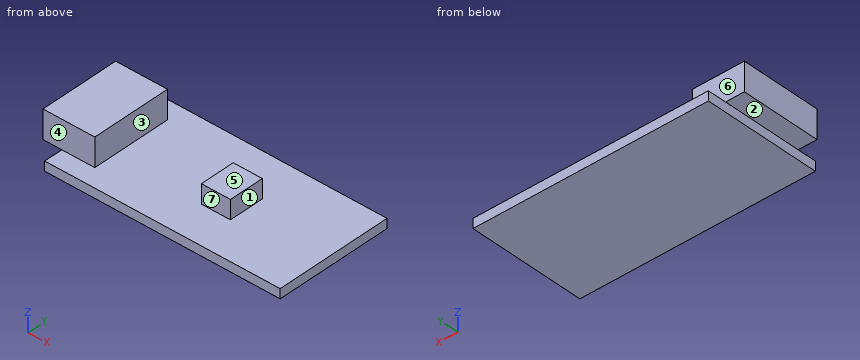
```python
from build123d import *

# Parameters (mm, degrees)
SKIZZE1_W                       = 25
SKIZZE1_H                       = 12.5
SKIZZE1_W_2                     = 3.091607018
SKIZZE1_H_2                     = 3.725771618
AUFSATZ_LINEAR_AUSTRAGEN1_DEPTH = 1
SKIZZE1_2_W                     = 3.091607018
SKIZZE1_2_H                     = 3.725771618
AUFSATZ_LINEAR_AUSTRAGEN2_DEPTH = 3
SKIZZE2_W                       = 5.5
SKIZZE2_H                       = 8.5
AUFSATZ_LINEAR_AUSTRAGEN3_DEPTH = 3


with BuildPart() as part:
    # Skizze1 → Aufsatz-Linear austragen1 (new body)
    with BuildSketch(Plane.XY):
        with Locations((12.5, 6.25)):
            Rectangle(SKIZZE1_W, SKIZZE1_H)
        with Locations((14.475260973, 5.942942992)):
            Rectangle(SKIZZE1_W_2, SKIZZE1_H_2, mode=Mode.SUBTRACT)
    extrude(amount=AUFSATZ_LINEAR_AUSTRAGEN1_DEPTH)

    # Skizze1<2> → Aufsatz-Linear austragen2 (add)
    with BuildSketch(Plane.XY):
        with Locations((14.475260973, 5.942942992)):
            Rectangle(SKIZZE1_2_W, SKIZZE1_2_H)
    extrude(amount=AUFSATZ_LINEAR_AUSTRAGEN2_DEPTH)

    # Skizze2 → Aufsatz-Linear austragen3 (add)
    with BuildSketch(Plane.XY.offset(1)):
        with Locations((0.75, 6.25)):
            Rectangle(SKIZZE2_W, SKIZZE2_H)
    extrude(amount=AUFSATZ_LINEAR_AUSTRAGEN3_DEPTH)


solid = part.part
```
Verification items for the finished model (mm, model axes). Face numbers are marked on the shaded views. A direction names the side the tool comes from. Coordinates: 2 decimals unless noted, no trailing zeros. Order: outer loops, then holes, each group sorted by start corner. A loop starts at its lowest first (then second) coordinate and runs counter-clockwise, first axis right, second up. Notation, with made-up numbers: (34.25, 30) - (43.25, 30) arc R30 cw to (43.25, 58) - close; hole circle Ø4 at (15, 16). An arc over 180 degrees is marked (long way). Return JSON: item names as keys, results as strings.
(1) Mould release check, pull along X, two halves, no side actions. Record for the marked faces 1, 2 and 3: pulls with the +X half, pulls with the -X half, needs draft (parallel to the pull), parting line crosses it, or undercut.
Filled sheet:
{"face 1": "pulls with the +X half", "face 2": "needs draft", "face 3": "undercut"}
(2) Thickness scan on line 1 along Z through (x, y) = (22.75, 10.5); line 2 along X through (y, z) = (6.5, 2.5); line 3 along Z through (x, y) = (14.25, 4.5). Record the ranges inside material, lowest first.
Filled sheet:
{"line 1": "z = 0 to 1", "line 2": "x = -2 to 3.5, 12.93 to 16.02", "line 3": "z = 0 to 3"}
(3) Section check B-B, the plane y = 9. Record the cut outline in (x, z), and give its area (3 significant figures).
Filled sheet:
{"outline": "(-2, 1) - (0, 1) - (0, 0) - (25, 0) - (25, 1) - (3.5, 1) - (3.5, 4) - (-2, 4) - close", "area": "41.5 mm^2"}
(4) Section check C-C, the plane x = 14.5. Record the cut outline in (y, z), and give its area (3 significant figures).
Filled sheet:
{"outline": "(0, 0) - (12.5, 0) - (12.5, 1) - (7.81, 1) - (7.81, 3) - (4.08, 3) - (4.08, 1) - (0, 1) - close", "area": "20.0 mm^2"}
(5) Access from +Z, -Z, +X, -X, +Y, -Y to the whole of each face (thin tool, end or side, straight path). Record for the marked faces 4, 5, 6 and 7.
Filled sheet:
{"face 4": "+Z, +X, -X, -Y", "face 5": "+Z, +X, +Y, -Y", "face 6": "+Z, +X, -X, +Y", "face 7": "+Z, +X, -Y"}
(6) Section check A-A, the plane z = 1.4. Record the cut outline in (x, y).
Filled sheet:
{"outline": "(-2, 2) - (3.5, 2) - (3.5, 10.5) - (-2, 10.5) - close; (12.93, 4.08) - (16.02, 4.08) - (16.02, 7.81) - (12.93, 7.81) - close"}
(7) Section check D-D, the plane z = 3.55. Record the cut outline in (x, y), and give its area (4 significant figures).
Filled sheet:
{"outline": "(-2, 2) - (3.5, 2) - (3.5, 10.5) - (-2, 10.5) - close", "area": "46.75 mm^2"}
(8) Go/stop test with flat-tipped pins: pin 1 (6 mm diameter, centred on x = 17.5, y = 6, fed in from -Z); pin 2 (0.6 mm diameter, centred on x = -0.5, y = 7, fed in from -Z); pin 3 (3.5 mm diameter, centred on x = 14, y = 5.5, fed in from +Z); pin 4 (1.5 mm diameter, centred on x = 0.5, z = 2, fed in from +Y). Record where each tip stops, or that it passes through.
Filled sheet:
{"pin 1": "stops at z = 0", "pin 2": "stops at z = 1", "pin 3": "stops at z = 3", "pin 4": "stops at y = 10.5"}
